Build history of the part. All positions in model axes, mm. Coordinates: 2 decimals unless noted, no trailing zeros. Order: outer loops, then holes, each group sorted by start corner. A loop starts at its lowest first (then second) coordinate and runs counter-clockwise, first axis right, second up. Notation, with made-up numbers: M -10,53.25 L 34,53.25 A18 cw 34,77.25 Z; hole C 89.5,73.5 d3. An arc over 180 degrees is marked long. Write item = value, one per line. Start each with the question number.
Q1. Band-saw the part on C-C on y = -3.75. Write the cut outline in (x, z), plus the area to 3 significant figures.
Q2. Pull direction X, two halves, no side cores. Call faces 1 (the face through (0.45, -7.89, -1.43)), 2 (the face through (0, -16, 0)), 3 (the face through (0, 1.5, 0)): released by +X, released by -X, zero draft, split by the parting line, or undercut.
Q3. Pin check, flat tips, straight feed: P1, Ø0.6, axis at x = -1.5, y = 2, coming from the +Z side; P2, Ø0.6, axis at y = 1.5, z = 1.5, coming from the -X side; P3, Ø2, axis at x = 2, y = -7, coming from the -Z side. Stop position of each tip, or through.
Q4. Band-saw the part on B-B on z = 0. Write the cut outline in (x, y), plus the area to 3 significant figures.
Q5. Drill centre lines: probe 1 along Y at (x, z) = (-0.45, -0.1); probe 2 along X at (y, z) = (-8, 0.1); probe 3 along Y at (x, z) = (0.65, 1.5). Where is each one in solid material? Low to high.
Q6. Band-saw the part on A-A on x = 0. Write the cut outline in (y, z).
```python
from build123d import *

# Parameters (mm, degrees)
FILLET2_R           = 0.8
SKETCH3_W           = 0.9
SKETCH3_H           = 3.2
CUT_EXTRUDE1_DEPTH  = 0.5
SKETCH4_W           = 3.2
SKETCH4_H           = 0.9
CUT_EXTRUDE2_DEPTH  = 4.840572939
FILLET1_R           = 0.6
SKETCH2_R           = 1.5
BOSS_EXTRUDE1_DEPTH = 16


with BuildPart() as part:
    # Sketch1 → Revolve1 (revolve)
    with BuildSketch(Plane(origin=(0, 0, 0), x_dir=(0, 0, -1), z_dir=(1, 0, 0))):
        with BuildLine():
            Line((0, 2), (0, 0))
            Line((0, 0), (2.5, 0))
            ThreePointArc((2.5, 0), (1.914213562, 1.414213562), (0.5, 2))
            Line((0.5, 2), (0, 2))
        make_face()
        with BuildLine():
            ThreePointArc((0.5, 2), (1.914213562, 1.414213562), (2.5, 0))
            Line((2.5, 0), (2.5, 2))
            Line((2.5, 2), (0.5, 2))
        make_face()
    revolve(axis=Axis((0, 0, 0), (0, 1, 0)))

    # Fillet2
    fillet2_edges = [part.edges().sort_by_distance(p)[0] for p in [
        (0, 2, 2.5),
        (0, 0, 2.5),
    ]]
    fillet(fillet2_edges, radius=FILLET2_R)

    # Sketch3 → Cut-Extrude1 (cut)
    with BuildSketch(Plane(origin=(0, 2, 0), x_dir=(1, 0, 0), z_dir=(0, 1, 0))):
        Rectangle(SKETCH3_W, SKETCH3_H)
    extrude(amount=-CUT_EXTRUDE1_DEPTH, mode=Mode.SUBTRACT)

    # Sketch4 → Cut-Extrude2 (cut, through all)
    with BuildSketch(Plane(origin=(0, 1.5, 0), x_dir=(1, 0, 0), z_dir=(0, 1, 0))):
        Rectangle(SKETCH4_W, SKETCH4_H)
    extrude(amount=CUT_EXTRUDE2_DEPTH, mode=Mode.SUBTRACT)

    # Fillet1
    fillet1_edges = [part.edges().sort_by_distance(p)[0] for p in [
        (0.45, 1.75, -0.45),
        (0.45, 1.75, 0.45),
        (-0.45, 1.75, -0.45),
        (-0.45, 1.75, 0.45),
    ]]
    fillet(fillet1_edges, radius=FILLET1_R)

    # Sketch2 → Boss-Extrude1 (add)
    with BuildSketch(Plane.XZ):
        with Locations(Location((0, 0, 0), (0, 0, 270))):
            Circle(SKETCH2_R)
    extrude(amount=BOSS_EXTRUDE1_DEPTH)


solid = part.part
```
Recorded:
q1.outline = C 0,0 d3
q1.area = 7.07 mm2
q2.face_1 = split by the parting line
q2.face_2 = zero draft
q2.face_3 = undercut
q3.P1 = 1.85
q3.P2 = -2.16
q3.P3 = -1.12
q4.outline = M -2.5,0.8 A0.8 ccw -1.7,0 L -1.5,0 L -1.5,-16 L 1.5,-16 L 1.5,0 L 1.7,0 A0.8 ccw 2.5,0.8 L 2.5,1.2 A0.8 ccw 1.7,2 L 1.6,2 L 1.6,1.5 L -1.6,1.5 L -1.6,2 L -1.7,2 A0.8 ccw -2.5,1.2 Z
q4.area = 55.9 mm2
q5.probe_1 = -16 to 1.5
q5.probe_2 = -1.5 to 1.5
q5.probe_3 = 0 to 2
q6.outline = M -16,-1.5 L 0,-1.5 L 0,-1.7 A0.8 ccw 0.8,-2.5 L 1.2,-2.5 A0.8 ccw 2,-1.7 L 2,-1.6 L 1.5,-1.6 L 1.5,1.6 L 2,1.6 L 2,1.7 A0.8 ccw 1.2,2.5 L 0.8,2.5 A0.8 ccw 0,1.7 L 0,1.5 L -16,1.5 Z
